from build123d import *

# Parameters (mm, degrees)
SKETCH057_W         = 65
SKETCH057_H         = 55
PAD015_DEPTH        = 2
SKETCH058_R         = 1.75
HOLE023_DEPTH       = 25
SKETCH059_W         = 44
SKETCH059_H         = 28
PAD016_DEPTH        = 30
SKETCH060_W         = 40.4
SKETCH060_H         = 24.4
POCKET018_DEPTH     = 30
SKETCH061_W         = 20
SKETCH061_H         = 20
SKETCH061_W_2       = 40
POCKET019_DEPTH     = 28
SKETCH062_W         = 24
SKETCH062_H         = 22
POCKET020_DEPTH     = 50
SKETCH063_R         = 1.75
HOLE024_DEPTH       = 25
HOLE025_D           = 3.5
HOLE025_DEPTH       = 25
HOLE025_CSINK_D     = 8
HOLE025_CSINK_ANGLE = 90
HOLE025_TIPS_R      = 1.75
FILLET022_R         = 1
FILLET023_R         = 1


with BuildPart() as part:
    # Sketch057 → Pad015 (new body)
    with BuildSketch(Plane.XY):
        Rectangle(SKETCH057_W, SKETCH057_H)
    extrude(amount=PAD015_DEPTH)

    # Sketch058 (on Face6 of Pad015) → Hole023 (cut)
    with BuildSketch(Plane.XY.offset(2)):
        with Locations((25, 20)):
            Circle(SKETCH058_R)
        with Locations((25, -20)):
            Circle(SKETCH058_R)
    hole023 = extrude(amount=-HOLE023_DEPTH, mode=Mode.SUBTRACT)

    # Mirrored028: Hole023 across Sketch058 V_Axis
    add(hole023.mirror(Plane(origin=(0, 0, 2), x_dir=(0, 0, 1), z_dir=(1, 0, 0))), mode=Mode.SUBTRACT)

    # Sketch059 (on Face5 of Mirrored028) → Pad016 (join)
    with BuildSketch(Plane.XY.offset(2)):
        Rectangle(SKETCH059_W, SKETCH059_H)
    extrude(amount=PAD016_DEPTH)

    # Sketch060 (on Face15 of Pad016) → Pocket018 (cut)
    with BuildSketch(Plane.XY.offset(32)):
        Rectangle(SKETCH060_W, SKETCH060_H)
    extrude(amount=-POCKET018_DEPTH, mode=Mode.SUBTRACT)

    # Sketch061 (on Face15 of Pocket018) → Pocket019 (cut)
    with BuildSketch(Plane.XY.offset(32)):
        with Locations((0, 10)):
            Rectangle(SKETCH061_W, SKETCH061_H)
        with Locations((20, 0)):
            Rectangle(SKETCH061_W_2, SKETCH061_H)
    extrude(amount=-POCKET019_DEPTH, mode=Mode.SUBTRACT)

    # Sketch062 (on Face11 of Pocket019) → Pocket020 (cut)
    with BuildSketch(Plane(origin=(-22, 0, 0), x_dir=(0, -1, 0), z_dir=(-1, 0, 0))):
        with Locations((0, 14)):
            Rectangle(SKETCH062_W, SKETCH062_H)
    extrude(amount=-POCKET020_DEPTH, mode=Mode.SUBTRACT)

    # Sketch063 (on Face35 of Pocket020) → Hole024 (cut)
    with BuildSketch(Plane.XY.offset(2)):
        with Locations((-16.2, 8.2)):
            Circle(SKETCH063_R)
        with Locations((-16.2, -8.2)):
            Circle(SKETCH063_R)
    extrude(amount=-HOLE024_DEPTH, mode=Mode.SUBTRACT)

    # Hole025
    with Locations(Plane(origin=(0, 0, 0), x_dir=(1, 0, 0), z_dir=(0, 0, -1))):
        with Locations((-16.2, -8.2), (-16.2, 8.2)):
            CounterSinkHole(HOLE025_D / 2, HOLE025_CSINK_D / 2, depth=HOLE025_DEPTH, counter_sink_angle=HOLE025_CSINK_ANGLE)

    # Hole025 tips → Hole025 tip 1 section 0
    with BuildSketch(Plane(origin=(0, 0, 25), x_dir=(1, 0, 0), z_dir=(0, 0, -1)), mode=Mode.PRIVATE) as hole025_tip_1_s0:
        with Locations((-16.2, -8.2)):
            Circle(HOLE025_TIPS_R)
    loft([hole025_tip_1_s0.sketch, Vertex(-16.2, 8.2, 26.051506)], mode=Mode.SUBTRACT)

    # Hole025 tips → Hole025 tip 2 section 0
    with BuildSketch(Plane(origin=(0, 0, 25), x_dir=(1, 0, 0), z_dir=(0, 0, -1)), mode=Mode.PRIVATE) as hole025_tip_2_s0:
        with Locations((-16.2, 8.2)):
            Circle(HOLE025_TIPS_R)
    loft([hole025_tip_2_s0.sketch, Vertex(-16.2, -8.2, 26.051506)], mode=Mode.SUBTRACT)

    # Fillet022
    fillet022_edges = [part.edges().sort_by_distance(p)[0] for p in [
        (32.5, -27.5, 1),
        (32.5, 27.5, 1),
        (-32.5, -27.5, 1),
        (-32.5, 27.5, 1),
    ]]
    fillet(fillet022_edges, radius=FILLET022_R)

    # Fillet023
    fillet023_edges = [part.edges().sort_by_distance(p)[0] for p in [
        (22, 14, 17),
        (-22, 14, 17),
        (22, -14, 17),
        (-22, -14, 17),
    ]]
    fillet(fillet023_edges, radius=FILLET023_R)


solid = part.part
Part model, mm, in its own coordinate system. A direction names the side the tool comes from. Coordinates: 2 decimals unless noted, no trailing zeros. Loops run counter-clockwise (first coordinate to the right, second up) from the corner with the lowest first, then second, coordinate; pieces in that order, holes last. Notation, with made-up numbers: (33.25, 67) -> (63.25, 67) arc R12 cw to (63.25, 88) -> close; hole circle Ø8 at (35.25, -4). An arc over 180 degrees is marked (long way). Use a Markdown table: item, result. Add a question column.
Item 1: Which spindle directions (+Z, -Z, +X, -X, +Y, -Y) get a long thin tool onto all of the face, cutting with end or side? Do faces 4 (the flat face through (-21, 12, 14)), 5 (the flat face through (21, -10, 29)), 6 (the flat face through (0, 13, 4)), 7 (the flat face through (-14, 12.2, 17)). Say none if no direction does.
Item 2: Band-saw the part on C-C on y = -8.2. Write the cut outline in (x, z), plus the area to 3 significant figures.
Item 3: Probe probe 1 along Y at (x, z) = (-25, 0.85); probe 2 along Y at (x, z) = (14, 6); probe 3 along Y at (x, z) = (-5.5, 7). List the from-to ranges inside material, lowest first.
Item 4: Band-saw the part on A-A on z = 13.5. Write the cut outline in (x, y).
Item 5: Band-saw the part on B-B on x = -25. Write the cut outline in (y, z).
Item 6: Flat gauge pins, fed straight in: P1, Ø1, axis at x = 7.5, y = -20.5, coming from the +Z side; P2, Ø0.9, axis at x = 21.5, z = 29, coming from the -Y side; P3, Ø3, axis at x = 25, y = 20, coming from the -Z side; P4, Ø1.4, axis at y = 13, z = 20.5, coming from the -X side. Where does each tip first touch, or does it go through?
Item 7: Band-saw the part on D-D on z = 27.5. Write the cut outline in (x, y), plus the area to 3 significant figures.
Item 8: Pull direction Z, two halves, no side cores. Call faces 1 (the flat face through (-8.3, -12.4, 32)), 2 (the flat face through (0, 27.5, 1)), 3 (the flat face through (21, 11, 25)): +Z half, -Z half, draft (parallel to the pull), parting line (faces both ways), or undercut.
Geometry says:
| question | item | result |
|---|---|---|
| 1 | face 4 | +X, -X |
| 1 | face 5 | +Z, +X |
| 1 | face 6 | +Z, +Y |
| 1 | face 7 | +Z |
| 2 | outline | (-32.5, 0) -> (-20.2, 0) -> (-18.2, 2) -> (-20.2, 2) -> (-20.2, 3) -> (-22, 3) -> (-22, 2) -> (-32.5, 2) -> close; (-22, 25) -> (-20.2, 25) -> (-20.2, 32) -> (-22, 32) -> close; (-14.2, 2) -> (-12.2, 0) -> (32.5, 0) -> (32.5, 2) -> (22, 2) -> (22, 3) -> (20.2, 3) -> (20.2, 2) -> close |
| 2 | area | 134 mm² |
| 3 | probe 1 | -27.5 to -21.75, -18.25 to 18.25, 21.75 to 27.5 |
| 3 | probe 2 | -14 to -12.2, 12.2 to 14 |
| 3 | probe 3 | -14 to -12.2 |
| 4 | outline | (-22, -13) arc R1 ccw to (-21, -14) -> (21, -14) arc R1 ccw to (22, -13) -> (22, -12) -> (20.2, -12) -> (20.2, -12.2) -> (-20.2, -12.2) -> (-20.2, -12) -> (-22, -12) -> close; (-22, 12) -> (-20.2, 12) -> (-20.2, 12.2) -> (-10, 12.2) -> (-10, 14) -> (-21, 14) arc R1 ccw to (-22, 13) -> close; (10, 12.2) -> (20.2, 12.2) -> (20.2, 12) -> (22, 12) -> (22, 13) arc R1 ccw to (21, 14) -> (10, 14) -> close |
| 5 | outline | (-27.5, 0) -> (-21.75, 0) -> (-21.75, 2) -> (-27.5, 2) -> close; (-18.25, 0) -> (18.25, 0) -> (18.25, 2) -> (-18.25, 2) -> close; (21.75, 0) -> (27.5, 0) -> (27.5, 2) -> (21.75, 2) -> close |
| 6 | P1 | z = 2 |
| 6 | P2 | y = -14 |
| 6 | P3 | through |
| 6 | P4 | x = -22 |
| 7 | outline | (-22, -13) arc R1 ccw to (-21, -14) -> (21, -14) arc R1 ccw to (22, -13) -> (22, -10) -> (20.2, -10) -> (20.2, -12.2) -> (-20.2, -12.2) -> (-20.2, 12.2) -> (-10, 12.2) -> (-10, 14) -> (-21, 14) arc R1 ccw to (-22, 13) -> close; (10, 12.2) -> (20.2, 12.2) -> (20.2, 10) -> (22, 10) -> (22, 13) arc R1 ccw to (21, 14) -> (10, 14) -> close |
| 7 | area | 173 mm² |
| 8 | face 1 | +Z half |
| 8 | face 2 | draft |
| 8 | face 3 | undercut |
